```python
from build123d import *

# Parameters (mm, degrees)
SKETCH_1_R      = 3
EXTRUDE_1_DEPTH = 40
CHAMFER_1_SIZE  = 0.5


with BuildPart() as part:
    # ｽｹｯﾁ1 → ﾎﾞｽ - 押し出し1 (new, symmetric)
    with BuildSketch(Plane.XY):
        Circle(SKETCH_1_R)
    extrude(amount=EXTRUDE_1_DEPTH, both=True)

    # 面取り1
    chamfer_1_edges = [part.edges().sort_by_distance(p)[0] for p in [
        (-3, 0, -40),
        (-3, 0, 40),
    ]]
    chamfer(chamfer_1_edges, length=CHAMFER_1_SIZE)

    # ｽｹｯﾁ3 → M3 ねじ穴1 (revolve, cut)
    with BuildSketch(Plane(origin=(0, 0, 40), x_dir=(0, -1, 0), z_dir=(1, 0, 0))):
        Polygon((0, 0), (0, 9.251075774), (1.25, 8.5), (1.25, 0), align=None)
    hole_wizard_m3_1 = revolve(axis=Axis((0, 0, 46.35), (0, 0, -1)), mode=Mode.SUBTRACT)

    # ﾐﾗｰ1: M3 ねじ穴1 across plane
    add(hole_wizard_m3_1.mirror(Plane.XY), mode=Mode.SUBTRACT)


solid = part.part
```
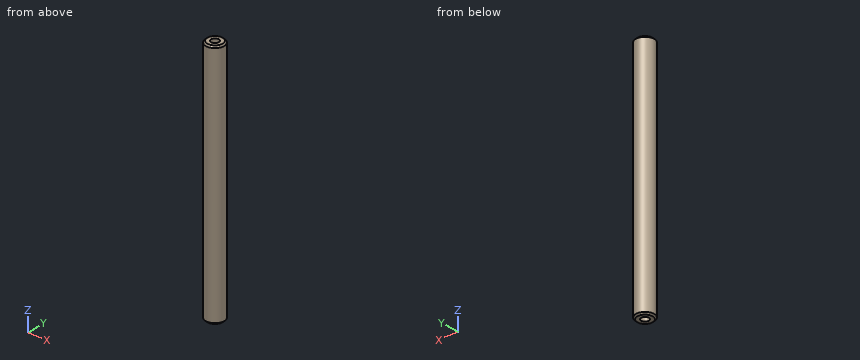
For this review, take the finished solid that the model builds, in its own axes (mm). Coordinates: 2 decimals unless noted, no trailing zeros. Loops run counter-clockwise (first coordinate to the right, second up) from the corner with the lowest first, then second, coordinate; pieces in that order, holes last. Notation, with made-up numbers: (32, 74.5) -> (68, 74.5) arc R20 ccw to (68, 98.5) -> close; hole circle Ø9 at (-20.5, 52.25). An arc over 180 degrees is marked (long way). Return JSON: item names as keys, results as strings. Group by question number.
(1) Consider section A-A, the plane z = 27. Give the boundary of the cut face in (x, y).
(2) For pin 1 Ø1.5 at (x, z) = (-2, -7) entering from +Y; pin 2 Ø2 at (x, z) = (1.5, 14.5) entering from +Y; pin 3 Ø2 at (x, y) = (0, 0) entering from -Z, all flat-tipped, find the tip position at first contact; note any pin that passes through.
(3) To check wall thickness, follow L1, parallel to Y at x = 0, z = -36.25; L2, parallel to X at y = -0.15, z = 1; L3, parallel to Z at x = 2.35, y = -0.9. State the ranges of each line that lie inside material, in increasing order.
Results below:
{
 "1": {"outline": "circle Ø6 at (0, 0)"},
 "2": {"pin 1": "stops at y = 2.73", "pin 2": "stops at y = 2.96", "pin 3": "stops at z = -31.35"},
 "3": {"L1": "y = -3 to -1.25, 1.25 to 3", "L2": "x = -3 to 3", "L3": "z = -39.98 to 39.98"}
}
